Build history of the part. All positions in model axes, mm. Face numbers are marked on the shaded views. A direction names the side the tool comes from. Coordinates: 2 decimals unless noted, no trailing zeros. Order: outer loops, then holes, each group sorted by start corner. A loop starts at its lowest first (then second) coordinate and runs counter-clockwise, first axis right, second up. Notation, with made-up numbers: (86.5, -6.5) - (140.5, -6.5) arc R17 cw to (140.5, 11.5) - close; hole circle Ø3 at (67, 26.25). An arc over 180 degrees is marked (long way). Write each question's results on one line, items separated by ' | '.
from build123d import *

# Parameters (mm, degrees)
SKETCH1_W           = 32
SKETCH1_H           = 60
BOSS_EXTRUDE1_DEPTH = 2.5
SKETCH2_R           = 5
BOSS_EXTRUDE2_DEPTH = 50
SKETCH3_W           = 1
SKETCH3_H           = 60
BOSS_EXTRUDE3_DEPTH = 30


with BuildPart() as part:
    # Sketch1 → Boss-Extrude1 (new body, symmetric)
    with BuildSketch(Plane(origin=(0, 0, 0), x_dir=(1, 0, 0), z_dir=(0, 1, 0))):
        Rectangle(SKETCH1_W, SKETCH1_H)
    extrude(amount=BOSS_EXTRUDE1_DEPTH, both=True)

    # Sketch2 → Boss-Extrude2 (add)
    with BuildSketch(Plane.XZ.offset(2.5)):
        with Locations((0, 16)):
            Circle(SKETCH2_R)
        with Locations((0, -16)):
            Circle(SKETCH2_R)
    extrude(amount=BOSS_EXTRUDE2_DEPTH)

    # Sketch3 → Boss-Extrude3 (add)
    with BuildSketch(Plane(origin=(0, 2.5, 0), x_dir=(1, 0, 0), z_dir=(0, 1, 0))):
        with Locations((-15.5, 0)):
            Rectangle(SKETCH3_W, SKETCH3_H)
        with Locations((15.5, 0)):
            Rectangle(SKETCH3_W, SKETCH3_H)
    extrude(amount=BOSS_EXTRUDE3_DEPTH)


solid = part.part
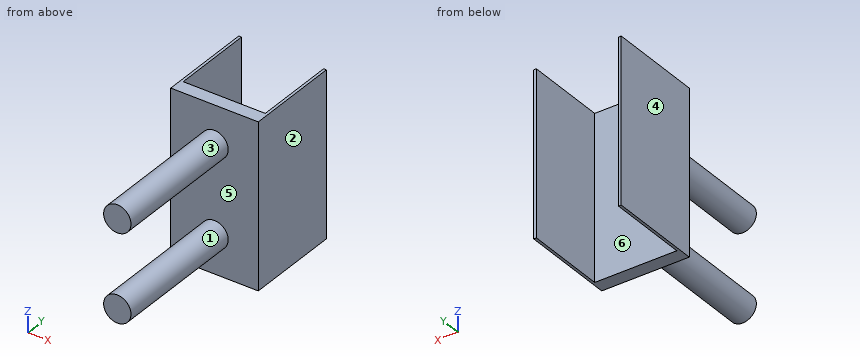
1. Probe line 1 (X direction, y = 23, z = -21); line 2 (Y direction, x = 9, z = 25); line 3 (Y direction, x = 2.5, z = 13.5). List the from-to ranges inside material, lowest first.
Solved:
line 1: x = -16 to -15, 15 to 16 | line 2: y = -2.5 to 2.5 | line 3: y = -52.5 to 2.5
2. Band-saw the part on D-D on z = -16. Give the cut face in (x, y).
Solved:
outline: (-16, -2.5) - (-5, -2.5) - (-5, -52.5) - (5, -52.5) - (5, -2.5) - (16, -2.5) - (16, 32.5) - (15, 32.5) - (15, 2.5) - (-15, 2.5) - (-15, 32.5) - (-16, 32.5) - close
3. Drop flat-ended pins along their axis: pin 1 Ø9 at (x, z) = (-7, 10) entering from +Y; pin 2 Ø2 at (y, z) = (-25.5, -19.5) entering from -X; pin 3 Ø12 at (x, y) = (1.5, -32.5) entering from +Z. Give the stop position or say it passes through.
Solved:
pin 1: stops at y = 2.5 | pin 2: stops at x = -4.33 | pin 3: stops at z = 21
4. Two-plate mould, pull along Z, no slides. Class the marked faces 1, 2 and 3: +Z half, -Z half, draft (parallel to the pull), parting line (faces both ways), or undercut.
Solved:
face 1: undercut | face 2: draft | face 3: undercut
5. Band-saw the part on A-A on z = 0.5. Give the cut face in (x, y), then the cut area to 3 significant figures.
Solved:
outline: (-16, -2.5) - (16, -2.5) - (16, 32.5) - (15, 32.5) - (15, 2.5) - (-15, 2.5) - (-15, 32.5) - (-16, 32.5) - close | area: 220 mm2
6. Tool access for the marked faces 4, 5 and 6: list every direction of +Z, -Z, +X, -X, +Y, -Y with a clear straight run to the whole face (end or side of a thin tool).
Solved:
face 4: +Z, -Z, -X, +Y, -Y | face 5: -Y | face 6: +Z, -Z, +Y
7. Band-saw the part on C-C on y = -31. Give the cut face in (x, z), then the cut area to 3 significant figures.
Solved:
outline: circle Ø10 at (0, -16); circle Ø10 at (0, 16) | area: 157 mm2
8. Band-saw the part on B-B on x = 0. Give the cut face in (y, z).
Solved:
outline: (-52.5, -21) - (-2.5, -21) - (-2.5, -30) - (2.5, -30) - (2.5, 30) - (-2.5, 30) - (-2.5, 21) - (-52.5, 21) - (-52.5, 11) - (-2.5, 11) - (-2.5, -11) - (-52.5, -11) - close
